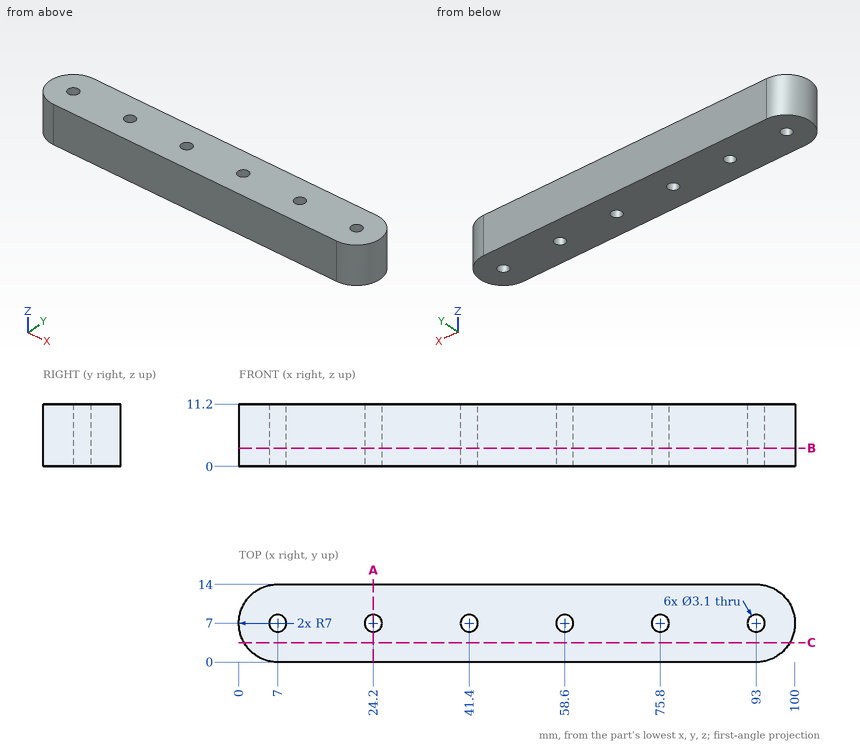
For this review, use the dimensioned drawing (mm, ordinates from the lowest corner) and the shaded views. Give positions to 0.01 mm unless a question says otherwise; leave off trailing zeros. Order: outer loops, then holes, each group sorted by start corner. A loop starts at its lowest first (then second) coordinate and runs counter-clockwise, first axis right, second up. Notation, with made-up numbers: (54, 56.5) -> (108, 56.5) arc R13 cw to (108, 64.5) -> close; hole circle Ø11 at (6.5, 42). An arc over 180 degrees is marked (long way). Write item = value, one per line. Start each with the question number.
(1) For L1, parallel to Y at x = 24.2, z = 8.5; L2, parallel to Y at x = 60, z = 2.5; L3, parallel to X at y = 9.5, z = 2.5, list the stretches that pass through material, from the lowest coordinate up. Write a range as from..to.
(2) Take a section at C-C (y = 3.5). Write out the cut boundary in (x, z).
(3) Take a section at B-B (z = 3.25). Write out the cut boundary in (x, y).
(4) For pin 1 Ø3 at (y, z) = (9, 10) entering from -X, flat-tipped, find the tip position at first contact; note if it passes through.
(5) Take a section at A-A (x = 24.2). Write out the cut boundary in (y, z), plus the area to 3 significant figures.
Returned:
q1.L1 = 0..5.45, 8.55..14
q1.L2 = 0..6.33, 7.67..14
q1.L3 = 0.46..99.54
q2.outline = (0.94, 0) -> (99.06, 0) -> (99.06, 11.2) -> (0.94, 11.2) -> close
q3.outline = (7, 0) -> (93, 0) arc R7 ccw to (93, 14) -> (7, 14) arc R7 ccw to start; hole circle Ø3.1 at (7, 7); hole circle Ø3.1 at (24.2, 7); hole circle Ø3.1 at (41.4, 7); hole circle Ø3.1 at (58.6, 7); hole circle Ø3.1 at (75.8, 7); hole circle Ø3.1 at (93, 7)
q4.pin_1 = 0.02
q5.outline = (0, 0) -> (5.45, 0) -> (5.45, 11.2) -> (0, 11.2) -> close; (8.55, 0) -> (14, 0) -> (14, 11.2) -> (8.55, 11.2) -> close
q5.area = 122 mm²
